Can you work these out from the model? Positions are in its coordinate system, mm. A direction names the side the tool comes from. Coordinates: 2 decimals unless noted, no trailing zeros. Loops run counter-clockwise (first coordinate to the right, second up) from the corner with the lowest first, then second, coordinate; pieces in that order, holes last.
Autodesk Inventor part; units mm, degrees
ref_plane "YZ Plane" through (0, 0, 0) normal (1, 0, 0) x (0, 1, 0)
ref_plane "XZ Plane" through (0, 0, 0) normal (0, 1, 0) x (-1, 0, 0)
ref_plane "XY Plane" through (0, 0, 0) normal (0, 0, 1) x (1, 0, 0)
sketch "Sketch1" plane through (0, 0, 0) normal (1, 0, 0) x (0, 1, 0)
  line L0 (180, 100) -> (-180, 100)
  line L1 (-180, 100) -> (-180, -100)
  line L2 (-180, -100) -> (180, -100)
  line L3 (180, -100) -> (180, 100)
  line L4 (180, 100) -> (-180, -100) construction
  line L5 (-180, 100) -> (180, -100) construction
  point P0 (0, 0)
  dimension "d0" = 360
  dimension "d1" = 200
extrude "Extrusion1" add sketch "Sketch1" along normal blind 3
sketch "Sketch7" plane through (3, 0, 0) normal (1, 0, 0) x (0, 0, -1)
  line L0 (1.5, 50) -> (-1.5, 50)
  line L1 (-1.5, 50) -> (-1.5, -50)
  line L2 (-1.5, -50) -> (1.5, -50)
  line L3 (1.5, -50) -> (1.5, 50)
  line L4 (1.5, 50) -> (-1.5, -50) construction
  line L5 (-1.5, 50) -> (1.5, -50) construction
  point P0 (0, 0)
  dimension "d69" = 3
  dimension "d70" = 100
extrude "Extrusion10" add sketch "Sketch7" along normal blind 24
sketch "Sketch8" plane through (3, -50, 1.5) normal (0, 0, 1) x (1, 0, 0)
  circle A0 centre (13, 75) radius 1.5
  circle A1 centre (13, 50) radius 1.5
  circle A2 centre (13, 25) radius 1.5
  line L0 (0, 100) -> (24, 100)
  line L1 (0, 0) -> (24, 0)
  line L2 (24, 100) -> (24, 0)
  line L3 (0, 230) -> (0, -130)
  point P0 (-3, 50)
  dimension "d73" = 3
  dimension "d74" = 3
  dimension "d75" = 3
  dimension "d76" = 25
  dimension "d77" = 25
  dimension "d78" = 25
  dimension "d87" = 25
  dimension "d88" = 11
  dimension "d89" = 11
  dimension "d90" = 11
extrude "Extrusion11" cut sketch "Sketch8" against normal blind 25 contours A0 | A1 | A2
properties part number "rightside"
Item 1: On a 3-axis mill with a long thin cutter (end or side, diameter ignored), from which of +Z, -Z, +X, -X, +Y, -Y can I reach the whole of each face in a straight line? I mean faces 1 (the face through (0, -3, 1)), 2 (the face through (12, -1, -1.5)), 3 (the face through (12, 1, 1.5)). Say none if no direction works.
Results are:
face 1: +Z, -Z, -X, +Y, -Y
face 2: -Z, +X, +Y, -Y
face 3: +Z, +X, +Y, -Y
Item 2: Suppose I cut it at C-C, the plane z = 45. Please give me the cut outline in (x, y), plus the area to 3 significant figures.
Results are:
outline: (0, -180) - (3, -180) - (3, 180) - (0, 180) - close
area: 1,080 mm2
Item 3: I'm going to push flat-ended pins straight in: P1, Ø3, axis at y = 31.5, z = 15, coming from the +X side; P2, Ø10, axis at x = 21.5, z = -5.5, coming from the +Y side; P3, Ø1.5, axis at x = 9.5, z = 0.5, coming from the -Y side. Where does each tip first touch, or does it pass through?
Results are:
P1: stops at x = 3
P2: stops at y = 50
P3: stops at y = -50
Item 4: I need wall thicknesses on line 1 along Y through (x, z) = (16, -0.45); line 2 along X through (y, z) = (-78.5, 7); line 3 along Y through (x, z) = (13.5, 0.5). Which ranges of each line are inside material? Lowest first, please.
Results are:
line 1: y = -50 to -26.5, -23.5 to -1.5, 1.5 to 23.5, 26.5 to 50
line 2: x = 0 to 3
line 3: y = -50 to 50
Item 5: Suppose I cut it at B-B, the plane x = 10.5. Please give me the cut outline in (y, z).
Results are:
outline: (-50, -1.5) - (50, -1.5) - (50, 1.5) - (-50, 1.5) - close
Item 6: Suppose I cut it at A-A, the plane y = 12. Please give me the cut outline in (x, z), plus the area to 3 significant figures.
Results are:
outline: (0, -100) - (3, -100) - (3, -1.5) - (27, -1.5) - (27, 1.5) - (3, 1.5) - (3, 100) - (0, 100) - close
area: 672 mm2
